Job drawing, mm, ordinate dimensions from the low corner. One solid piece. A direction names the side the tool comes from. Coordinates: 2 decimals unless noted, no trailing zeros. Use a Markdown table: item, result. Add a question column.
1) Drop flat-ended pins along their axis: P1, Ø3, axis at x = 7.5, y = 3.5, coming from the +Z side; P2, Ø1.5, axis at x = 42.5, y = 4.5, coming from the -Z side; P3, Ø1, axis at y = 3.5, z = 6.5, coming from the +X side. Give the stop position or say it passes through.
2) Tool access for the marked faces 1 and 2: list every direction of +Z, -Z, +X, -X, +Y, -Y with a clear straight run to the whole face (end or side of a thin tool).
3) Probe probe 1 along X at (y, z) = (8.75, 25.5) (1 decimal); probe 2 along Z at (x, y) = (25, 0.5) (1 decimal). List the from-to ranges inside material, lowest first. Write a range as [from, to].
4) Band-saw the part on C-C (y = 3). Give the number of separate pieces and of enclosed holes in the cut face, plus the area to 3 significant figures.
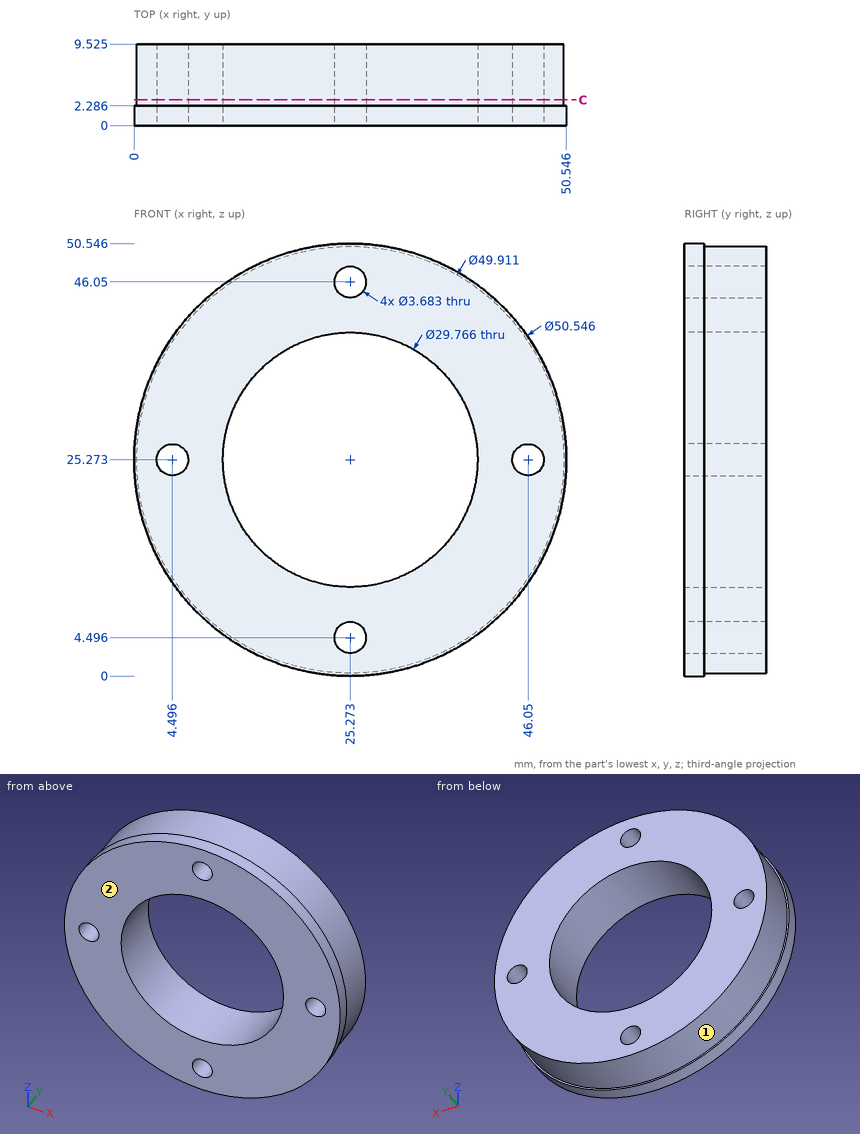
Answer block:
| question | item | result |
|---|---|---|
| 1 | P1 | z = 44.19 |
| 1 | P2 | z = 6.53 |
| 1 | P3 | x = 42.27 |
| 2 | face 1 | +Y |
| 2 | face 2 | +Z, -Z, +X, -X, -Y |
| 3 | probe 1 | [0.3, 2.7], [6.3, 10.4], [40.2, 44.2], [47.9, 50.2] |
| 3 | probe 2 | [0, 2.7], [6.3, 10.4], [40.2, 44.2], [47.9, 50.5] |
| 4 | separate pieces | 1 |
| 4 | enclosed holes | 5 |
| 4 | area | 1,220 mm2 |
